For this review, take the finished solid that the model builds, in its own axes (mm). A direction names the side the tool comes from. Round coordinates to 2 decimals unless told otherwise and drop trailing zeros. Order: outer loops, then holes, each group sorted by start corner. A loop starts at its lowest first (then second) coordinate and runs counter-clockwise, first axis right, second up. Notation, with made-up numbers: M 88.5,89 L 115.5,89 A19 ccw 115.5,117 Z; hole C -35.5,44.25 d11. An arc over 180 degrees is marked long. Write item = value, one per line. Start each with the question number.
from build123d import *

# Parameters (mm, degrees)
F0_R      = 31
F0_R_2    = 17.5
F1_DEPTH  = 10
F2_R      = 26
F3_DEPTH  = 5
F3_FACE_R = 17.5
F4_DEPTH  = 25.4


with BuildPart() as f1:
    # F0 (on Front) → F1 (new body)
    with BuildSketch(Plane.XZ):
        Circle(F0_R)
        Circle(F0_R_2, mode=Mode.SUBTRACT)
    extrude(amount=F1_DEPTH)

    # F2 (on face) → F3 (join)
    with BuildSketch(Plane.XZ.offset(10)):
        Circle(F2_R)
    extrude(amount=F3_DEPTH)

    # F3_face (on face) → F4 (cut)
    with BuildSketch(Plane(origin=(0, -10, 0), x_dir=(1, 0, 0), z_dir=(0, 1, 0))):
        Circle(F3_FACE_R)
    extrude(amount=-F4_DEPTH, mode=Mode.SUBTRACT)


solid = f1.part
(1) We need section A-A, the plane x = 0. Write out the cut boundary in (y, z), then the cut area to 3 significant figures.
(2) For line 1 along Z through (x, y) = (0, -8.75); line 2 along X through (y, z) = (-9.25, 0.5); line 3 along Z through (x, y) = (0, -11.5), list the stretches that pass through material, from the lowest coordinate up.
(3) We need section C-C, the plane y = -1.75. Write out the cut boundary in (x, z).
(4) For faces 4 (the flat face through (-16, -10, -21)), 5 (the flat face through (5, -15, -17)), list the 3-axis set-ups (+Z, -Z, +X, -X, +Y, -Y) from which the entire face can be reached by the end or side of a thin tool; tool diameter is ignored.
(5) We need section B-B, the plane z = 0. Write out the cut boundary in (x, y).
(6) We need section D-D, the plane x = -23. Write out the cut boundary in (y, z).
(7) Insertion check: pin 1 (3 mm diameter, centred on y = -7, z = 23.5, fed in from +X); pin 2 (1 mm diameter, centred on x = 14.5, y = -5.5, fed in from -Z); pin 3 (1 mm diameter, centred on y = -9.5, z = 23.5, fed in from +X); pin 4 (5 mm diameter, centred on x = 12.5, z = 3, fed in from -Y). Each pin has a flat end and moves straight along its axis. Give the tip position at first contact, or say it passes through.
(8) Draft analysis for pull direction X (two halves, no side actions). For faces 1 (the cylindrical face through (-13.887, -7.395, 10.648)), 2 (the flat face through (13, 0, -13)), 3 (the cylindrical face through (-4.036, -4.93, 30.736)), state which applies: released by +X, released by -X, zero draft, split by the parting line, or undercut.
Values:
q1.outline = M -15,-26 L -10,-26 L -10,-31 L 0,-31 L 0,-17.5 L -15,-17.5 Z; M -15,17.5 L 0,17.5 L 0,31 L -10,31 L -10,26 L -15,26 Z
q1.area = 355 mm²
q2.line_1 = -31 to -17.5, 17.5 to 31
q2.line_2 = -31 to -17.49, 17.49 to 31
q2.line_3 = -26 to -17.5, 17.5 to 26
q3.outline = C 0,0 d62; hole C 0,0 d35
q4.face_4 = -Y
q4.face_5 = +Z, -Z, +X, -X, -Y
q5.outline = M -31,-10 L -26,-10 L -26,-15 L -17.5,-15 L -17.5,0 L -31,0 Z; M 17.5,-15 L 26,-15 L 26,-10 L 31,-10 L 31,0 L 17.5,0 Z
q6.outline = M -15,-12.12 L -10,-12.12 L -10,-20.78 L 0,-20.78 L 0,20.78 L -10,20.78 L -10,12.12 L -15,12.12 Z
q7.pin_1 = 21.84
q7.pin_2 = -27.66
q7.pin_3 = 20.78
q7.pin_4 = through
q8.face_1 = undercut
q8.face_2 = zero draft
q8.face_3 = split by the parting line
